from build123d import *

# Parameters (mm, degrees)
SKETCH1_R           = 6
SKETCH1_R_2         = 3.5
BOSS_EXTRUDE1_DEPTH = 30
SKETCH3_W           = 2
SKETCH3_H           = 8
CUT_EXTRUDE1_DEPTH  = 1


with BuildPart() as part:
    # Sketch1 → Boss-Extrude1 (new body)
    with BuildSketch(Plane.XY):
        Circle(SKETCH1_R)
        Circle(SKETCH1_R_2, mode=Mode.SUBTRACT)
    extrude(amount=-BOSS_EXTRUDE1_DEPTH)

    # Sketch3 → Cut-Extrude1 (cut)
    with BuildSketch(Plane(origin=(0, 6, 0), x_dir=(1, 0, 0), z_dir=(0, 1, 0))):
        with Locations((0, 6)):
            Rectangle(SKETCH3_W, SKETCH3_H)
    extrude(amount=-CUT_EXTRUDE1_DEPTH, mode=Mode.SUBTRACT)


solid = part.part
CAD build for the part. Positions are in the model's coordinates, mm. A direction names the side the tool comes from. Round coordinates to 2 decimals unless told otherwise and drop trailing zeros. Loops run counter-clockwise (first coordinate to the right, second up) from the corner with the lowest first, then second, coordinate; pieces in that order, holes last.
(1) Wall check: line 1 along Y through (x, z) = (0, -14); line 2 along Y through (x, z) = (0, -5.75); line 3 along X through (y, z) = (2.5, -5.75). Give the ranges that are in metal, low to high.
(2) Two-plate mould, pull along X, no slides. Class faces 3 (the flat face through (-1, 5.5, -5.9)), 4 (the cylindrical face through (-1.301, -5.857, -14.79)), 5 (the flat face through (3, -3, -30)): +X half, -X half, draft (parallel to the pull), parting line (faces both ways), or undercut.
(3) Cut at A-A (y = 0). Give the cut face in (x, z).
(4) Drop flat-ended pins along their axis: pin 1 (1.5 mm diameter, centred on x = -0.5, y = -3, fed in from +Z); pin 2 (0.7 mm diameter, centred on y = 5.5, z = -6, fed in from +X); pin 3 (4 mm diameter, centred on y = -4, z = -23.5, fed in from +X); pin 4 (6 mm diameter, centred on x = 3.5, z = -14, fed in from +Y). Give the stop position or say it passes through.
(5) Cut at D-D (x = 1.75). Give the cut face in (y, z).
(6) Cut at B-B (x = 0). Give the cut face in (y, z).
(7) Cut at C-C (z = -4.25). Give the cut face in (x, y).
(8) Which spindle directions (+Z, -Z, +X, -X, +Y, -Y) get a long thin tool onto all of the face, cutting with end or side? Do faces 1 (the flat face through (0, 5, -6)), 2 (the flat face through (3, -3, 0)). Say none if no direction does.
Findings below:
1. line 1: y = -6 to -3.5, 3.5 to 6
1. line 2: y = -6 to -3.5, 3.5 to 5
1. line 3: x = -5.45 to -2.45, 2.45 to 5.45
2. face 3: undercut
2. face 4: parting line
2. face 5: draft
3. outline: (-6, -30) - (-3.5, -30) - (-3.5, 0) - (-6, 0) - close; (3.5, -30) - (6, -30) - (6, 0) - (3.5, 0) - close
4. pin 1: stops at z = 0
4. pin 2: stops at x = 3.08
4. pin 3: stops at x = 5.66
4. pin 4: stops at y = 5.98
5. outline: (-5.74, -30) - (-3.03, -30) - (-3.03, 0) - (-5.74, 0) - close; (3.03, -30) - (5.74, -30) - (5.74, 0) - (3.03, 0) - close
6. outline: (-6, -30) - (-3.5, -30) - (-3.5, 0) - (-6, 0) - close; (3.5, -30) - (6, -30) - (6, -10) - (5, -10) - (5, -2) - (6, -2) - (6, 0) - (3.5, 0) - close
7. outline: (-1, 5) - (-1, 5.92) arc R6 ccw (long way) to (1, 5.92) - (1, 5) - close; hole circle Ø7 at (0, 0)
8. face 1: +Y
8. face 2: +Z, +X, -X, +Y, -Y
